from build123d import *

# Parameters (mm, degrees)
F1_DEPTH = 19.05
F2_SIZE  = 19.04999


# Not quite as in the source:
# - a fillet or chamfer is up to 0.001 mm smaller than in the source, because OpenCascade refuses the exact size


with BuildPart() as f1:
    # F0 (on Top) → F1 (new body)
    with BuildSketch(Plane.XY):
        Polygon((0, 1244.6), (0, 0), (647.7, 0), (647.7, 311.15), (936.6773304258, 596.9), (1374.8273304258, 596.9), (1374.8273304258, 1244.6), align=None)
    extrude(amount=F1_DEPTH)

    # F2 (size 19.05 in the source; OpenCascade refuses exactly that, so slightly less here)
    f2_edges = [f1.edges().sort_by_distance(p)[0] for p in [
        (647.7, 155.575, 0),
        (792.188665, 454.025, 0),
        (1155.75233, 596.9, 0),
        (323.85, 0, 0),
    ]]
    chamfer(f2_edges, length=F2_SIZE)


solid = f1.part
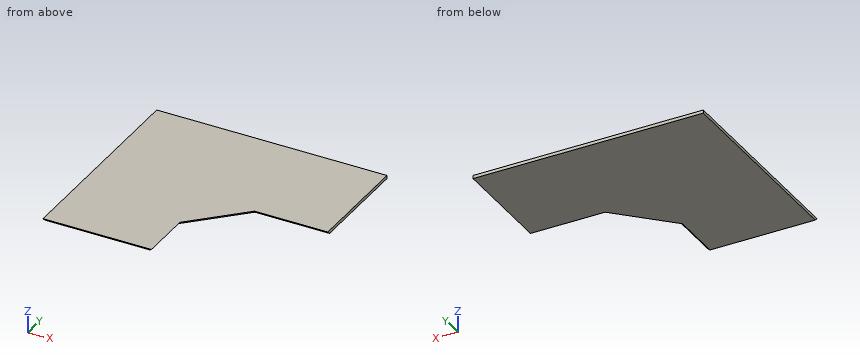
Geometry check sheet. Reference: the model listing, model coordinates, mm. Coordinates: 2 decimals unless noted, no trailing zeros. Order: outer loops, then holes, each group sorted by start corner. A loop starts at its lowest first (then second) coordinate and runs counter-clockwise, first axis right, second up. Notation, with made-up numbers: (69.5, 27.5) -> (94.5, 27.5) arc R30 ccw to (94.5, 61.5) -> close; hole circle Ø6 at (34, 77). An arc over 180 degrees is marked (long way). Use a Markdown table: item, result. Add a question column.
1. Cross-section at A-A (z = 14.25). Enter the section's corners in (x, y), and give its area (3 significant figures).
2. Material ranges on L1, parallel to Y at x = 527, z = 11.5; L2, parallel to Y at x = 1249.5, z = 7.75; L3, parallel to X at y = 528.5, z = 1, recorded low to high.
3. Go/stop test with flat-tipped pins: pin 1 Ø1.5 at (x, z) = (275, 16.5) entering from -Y; pin 2 Ø6 at (y, z) = (367.5, 10) entering from +X. Record where each tip stops, or that it passes through.
Filled sheet:
| question | item | result |
|---|---|---|
| 1 | outline | (0, 4.8) -> (642.9, 4.8) -> (642.9, 313.15) -> (934.7, 601.7) -> (1374.83, 601.7) -> (1374.83, 1244.6) -> (0, 1244.6) -> close |
| 1 | area | 1,310,000 mm2 |
| 2 | L1 | 7.55 to 1244.6 |
| 2 | L2 | 608.2 to 1244.6 |
| 2 | L3 | 0 to 841.83 |
| 3 | pin 1 | y = 1.8 |
| 3 | pin 2 | x = 697.05 |
